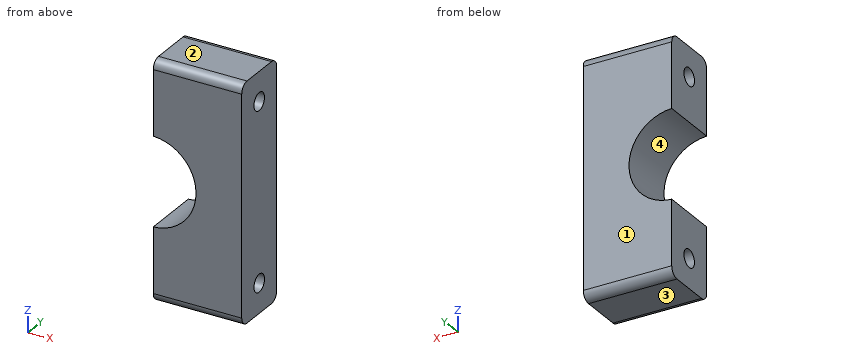
Autodesk Inventor part; units mm, degrees
ref_plane "YZ Plane" through (0, 0, 0) normal (1, 0, 0) x (0, 1, 0)
ref_plane "XZ Plane" through (0, 0, 0) normal (0, 1, 0) x (-1, 0, 0)
ref_plane "XY Plane" through (0, 0, 0) normal (0, 0, 1) x (1, 0, 0)
sketch "Sketch1" plane through (0, 0, 0) normal (0, 1, 0) x (-1, 0, 0)
  line L0 (-15, 40) -> (15, 40)
  line L1 (15, 40) -> (15, -40)
  line L2 (15, -40) -> (-15, -40)
  line L3 (-15, -40) -> (-15, 40)
  arc A0 (15, 14.9917) -> (15, -14.9917) centre (15.5, 0) ccw
  point P0 (0, 0)
  dimension "d0" = 80
  dimension "d1" = 30
  dimension "d2" = 40
  dimension "d3" = 15
  dimension "d4" = 30
  dimension "d22" = 0.5
extrude "Extrusion1" add sketch "Sketch1" along normal blind 20 contours L0 L1 A0 L2 L3
sketch "Sketch2" plane through (15, 0, 40) normal (1, 0, 0) x (0, 0, -1)
  line L0 (0, 0) -> (80, 0)
  line L1 (80, 0) -> (80, 20)
  line L2 (0, 20) -> (80, 20)
  line L3 (0, 0) -> (0, 20)
  point P0 (40, 0)
  point P1 (10, 10)
  point P2 (70, 10)
  dimension "d8" = 10
  dimension "d9" = 10
  dimension "d10" = 10
  dimension "d11" = 10
hole "Hole1" at (15, 10, 30) at (15, 10, -30) direction (-1, 0, 0) diameter 6 end through all
fillet "Fillet1" radius 3 4 edges at (0, 20, -40) (0, 20, 40) (0, 0, 40) (0, 0, -40)
properties part number "3DP_ASA_Balcony_Mounting_Clamp_Front"
The listing builds one solid part. Answer for the finished solid, in the listing's coordinates (mm). Face numbers are marked on the shaded views. Round coordinates to 2 decimals unless told otherwise and drop trailing zeros. Loops run counter-clockwise (first coordinate to the right, second up) from the corner with the lowest first, then second, coordinate; pieces in that order, holes last.
Q1. Find the intervals of material crossed by line 1 (Z direction, x = 5.75, y = 10.25); line 2 (Y direction, x = -2, z = 30); line 3 (Z direction, x = -4.75, y = 8.75), in increasing order.
Q2. Section B-B, the plane x = 3.75 is taken. Determine the outline of the cut face in (y, z), then the cut area to 3 significant figures.
Q3. Section C-C, the plane z = 30 is taken. Determine the outline of the cut face in (x, y), then the cut area to 3 significant figures.
Q4. For a pull along Z with two mould halves and no side action, classify the marked faces 1, 2, 3 and 4 as released by +Z, released by -Z, zero draft, split by the parting line, or undercut.
Q5. Given pin 1 Ø10 at (x, z) = (-2, 5.5) entering from +Y, flat-ended and moving along its own axis, determine where the tip first touches the part or whether it passes through.
Q6. Section A-A, the plane x = -3 is taken. Determine the outline of the cut face in (y, z).
Q7. Section D-D, the plane y = 10 is taken. Determine the outline of the cut face in (x, z), then the cut area to 3 significant figures.
Completed:
1. line 1: z = -40 to -32.99, -27.01 to 27.01, 32.99 to 40
1. line 2: y = 0 to 7, 13 to 20
1. line 3: z = -40 to -32.73, -27.27 to -10.46, 10.46 to 27.27, 32.73 to 40
2. outline: (0, -37) arc R3 ccw to (3, -40) - (17, -40) arc R3 ccw to (20, -37) - (20, 37) arc R3 ccw to (17, 40) - (3, 40) arc R3 ccw to (0, 37) - close; hole circle Ø6 at (10, -30); hole circle Ø6 at (10, 30)
2. area: 1,540 mm2
3. outline: (-15, 0) - (15, 0) - (15, 7) - (-15, 7) - close; (-15, 13) - (15, 13) - (15, 20) - (-15, 20) - close
3. area: 420 mm2
4. face 1: zero draft
4. face 2: released by +Z
4. face 3: released by -Z
4. face 4: undercut
5. pin 1: stops at y = 20
6. outline: (0, -37) arc R3 ccw to (3, -40) - (17, -40) arc R3 ccw to (20, -37) - (20, -8.29) - (0, -8.29) - close; (0, 8.29) - (20, 8.29) - (20, 37) arc R3 ccw to (17, 40) - (3, 40) arc R3 ccw to (0, 37) - close; hole circle Ø6 at (10, -30); hole circle Ø6 at (10, 30)
7. outline: (-15, -40) - (15, -40) - (15, -33) - (-15, -33) - close; (-15, -27) - (15, -27) - (15, 27) - (-15, 27) - (-15, 14.99) arc R15 cw to (-15, -14.99) - close; (-15, 33) - (15, 33) - (15, 40) - (-15, 40) - close
7. area: 1,700 mm2
